Geometry: final body of the model. Coordinates: model frame, mm. Face numbers are marked on the shaded views. A direction names the side the tool comes from. Give positions to 0.01 mm unless a question says otherwise; leave off trailing zeros. Loops run counter-clockwise (first coordinate to the right, second up) from the corner with the lowest first, then second, coordinate; pieces in that order, holes last. Notation, with made-up numbers: (-23, 52) -> (-3, 52) arc R9 ccw to (-3, 62) -> close; hole circle Ø5 at (66, 4). An arc over 180 degrees is marked (long way). One line per question, with ' | ' between items. Start each with the question number.
Item 1: Mould query, pull axis Y, two halves, no side actions, for the marked faces 6, 7, 8 and 9. Classes: released by +Y, released by -Y, zero draft, split by the parting line, or undercut.
Item 2: Section A-A on x = 9.75. Return loops of the section in (y, z).
Item 3: Section B-B on y = 21. Return loops of the section in (x, z).
Item 4: Section D-D on x = 16.25. Give the number of separate pieces and of enclosed holes in the cut face, then the cut area to 3 significant figures.
Item 5: Set-up query: the marked faces 1, 2, 3, 4 and 5. Return all of +Z, -Z, +X, -X, +Y, -Y with unobstructed straight access to the full face (end or side cutting, diameter ignored); none if empty.
Item 6: Material intervals for line 1 along Z through (x, y) = (19, -15.5); line 2 along Z through (x, y) = (13.25, 0); line 3 along X through (y, z) = (9.5, 17), sorted ascending. Write a range as [from, to].
Item 7: Section C-C on x = 13.5. Return loops of the section in (y, z).
Item 8: Pin query (flat end, axial travel): P1, Ø0.7, axis at x = 7, y = 6, coming from the +Z side; P2, Ø1.5, axis at x = 5, z = 8.5, coming from the +Y side; P3, Ø3, axis at x = 5, z = 8, coming from the +Y side. Return the tip coordinate at first contact, or that it passes through.
from build123d import *

# Parameters (mm, degrees)
SKETCH1_R                = 10
BOSS_EXTRUDE2_DEPTH      = 20
SKETCH5_R                = 12
BOSS_EXTRUDE3_DEPTH      = 12
BOSS_EXTRUDE4_DEPTH      = 5
FILLET2_R                = 3.175
F_5_0_5_DIAMETER_HOLE1_D = 5
FILLET1_START            = 15.0000001
FILLET1_DEPTH            = 4.9999999
FILLET1_START_2          = 11.8249999
FILLET1_2_DEPTH          = 3.1750001
CIRPATTERN6_START        = 11.8249999
CIRPATTERN6_OUTLINE_R    = 2.5
CIRPATTERN6_DEPTH        = 8.1750001
SKETCH2_R                = 5.5
SHAFT_HOLE_DEPTH         = 41.025175904
SKETCH3_W                = 4
SKETCH3_H                = 3.6
KEYWAY_DEPTH             = 41.025175904


with BuildPart() as part:
    # Sketch1 → Boss-Extrude2 (new body)
    with BuildSketch(Plane(origin=(0, 0, 0), x_dir=(0, 0, -1), z_dir=(1, 0, 0))):
        Circle(SKETCH1_R)
    extrude(amount=BOSS_EXTRUDE2_DEPTH)

    # Sketch5 → Boss-Extrude3 (add)
    with BuildSketch(Plane.ZY.offset(-20)):
        Circle(SKETCH5_R)
    extrude(amount=BOSS_EXTRUDE3_DEPTH)

    # Sketch6 → Boss-Extrude4 (add)
    with BuildSketch(Plane(origin=(20, 0, 0), x_dir=(0, 0, -1), z_dir=(1, 0, 0))):
        with BuildLine():
            Line((-5, 20), (-5, 0))
            Line((-5, 0), (5, 0))
            Line((5, 0), (5, 20))
            ThreePointArc((5, 20), (0, 25), (-5, 20))
        make_face()
    extrude(amount=-BOSS_EXTRUDE4_DEPTH)

    # Fillet2
    fillet2_edges = [part.edges().sort_by_distance(p)[0] for p in [
        (15, 12, 0),
    ]]
    fillet(fillet2_edges, radius=FILLET2_R)

    # Ø5.0 (5) Diameter Hole1 (through all)
    with Locations(Plane(origin=(20, 0, 0), x_dir=(0, 0, -1), z_dir=(1, 0, 0))):
        with Locations((0, 20)):
            Hole(F_5_0_5_DIAMETER_HOLE1_D / 2)

    # Fillet1: read off the stored shape, not the designer's step
    # Fillet1 outline → Fillet1 (add)
    with BuildSketch(Plane.YZ.offset(FILLET1_START)):
        with BuildLine():
            ThreePointArc((9.921567416, -6.75), (11.357927862, -5.464466094), (13.228756555, -5))
            Line((13.228756555, -5), (10.908712115, -5))
            ThreePointArc((10.908712115, -5), (10.451830526, -5.895696622), (9.921567416, -6.75))
        make_face()
        with BuildLine():
            ThreePointArc((13.228756555, 5), (11.357927862, 5.464466094), (9.921567416, 6.75))
            ThreePointArc((9.921567416, 6.75), (10.451830526, 5.895696622), (10.908712115, 5))
            Line((10.908712115, 5), (13.228756555, 5))
        make_face()
    extrude(amount=FILLET1_DEPTH)

    # Fillet1 2 outline → Fillet1 2 (add)
    with BuildSketch(Plane.YZ.offset(FILLET1_START_2)):
        with BuildLine():
            ThreePointArc((9.921567416, -6.75), (11.357927862, -5.464466094), (13.228756555, -5))
            Line((13.228756555, -5), (10.908712115, -5))
            ThreePointArc((10.908712115, -5), (10.451830526, -5.895696622), (9.921567416, -6.75))
        make_face()
        with BuildLine():
            ThreePointArc((13.228756555, 5), (11.357927862, 5.464466094), (9.921567416, 6.75))
            ThreePointArc((9.921567416, 6.75), (10.451830526, 5.895696622), (10.908712115, 5))
            Line((10.908712115, 5), (13.228756555, 5))
        make_face()
    extrude(amount=FILLET1_2_DEPTH)

    # Fillet1 3 outline → Fillet1 3 (revolve, cut)
    with BuildSketch(Plane.YX):
        with BuildLine():
            Line((15.175, 11.8249999), (15.175, 15))
            ThreePointArc((15.175, 15), (12.92993597, 14.07006403), (12, 11.825))
            Line((12, 11.825), (15.175, 11.8249999))
        make_face()
    revolve(axis=Axis((0, 0, 0), (1, 0, 0)), mode=Mode.SUBTRACT)

    # CirPattern6: read off the stored shape, not the designer's step
    # CirPattern6 outline → CirPattern6 (add)
    # profile 1 of 4: a face of its own
    with BuildSketch(Plane.YZ.offset(CIRPATTERN6_START)):
        with BuildLine():
            Line((8.843193172, 11.036210153), (10.935622469, 17.476045354))
            ThreePointArc((10.935622469, 17.476045354), (7.725424859, 23.776412907), (1.425057306, 20.566215298))
            Line((1.425057306, 20.566215298), (-0.667371991, 14.126380096))
            ThreePointArc((-0.667371991, 14.126380096), (-1.687223357, 12.490644193), (-3.353698542, 11.521836055))
            ThreePointArc((-3.353698542, 11.521836055), (3.708203933, 11.412678195), (9.485564428, 7.350106631))
            ThreePointArc((9.485564428, 7.350106631), (8.706808817, 9.113418416), (8.843193172, 11.036210153))
        make_face()
        with Locations((6.180339887, 19.021130326)):
            Circle(CIRPATTERN6_OUTLINE_R, mode=Mode.SUBTRACT)
    # profile 2 of 4: a face of its own
    with BuildSketch(Plane.YZ.offset(CIRPATTERN6_START)):
        with BuildLine():
            ThreePointArc((-11.994267104, 0.370886295), (-9.708203933, 7.053423027), (-4.059166198, 11.292615719))
            ThreePointArc((-4.059166198, 11.292615719), (-5.976824079, 11.096868429), (-7.763362606, 11.820752981))
            Line((-7.763362606, 11.820752981), (-13.241413626, 15.800790018))
            ThreePointArc((-13.241413626, 15.800790018), (-20.225424859, 14.694631307), (-19.119266149, 7.710620074))
            Line((-19.119266149, 7.710620074), (-13.641215129, 3.730583038))
            ThreePointArc((-13.641215129, 3.730583038), (-12.400689243, 2.255176559), (-11.994267104, 0.370886295))
        make_face()
        with Locations((-16.180339887, 11.755705046)):
            Circle(CIRPATTERN6_OUTLINE_R, mode=Mode.SUBTRACT)
    # profile 3 of 4: a face of its own
    with BuildSketch(Plane.YZ.offset(CIRPATTERN6_START)):
        with BuildLine():
            ThreePointArc((8.843193172, -11.036210153), (8.706808817, -9.113418416), (9.485564428, -7.350106631))
            ThreePointArc((9.485564428, -7.350106631), (3.708203933, -11.412678195), (-3.353698542, -11.521836055))
            ThreePointArc((-3.353698542, -11.521836055), (-1.687223357, -12.490644193), (-0.667371991, -14.126380096))
            Line((-0.667371991, -14.126380096), (1.425057306, -20.566215298))
            ThreePointArc((1.425057306, -20.566215298), (7.725424859, -23.776412907), (10.935622469, -17.476045354))
            Line((10.935622469, -17.476045354), (8.843193172, -11.036210153))
        make_face()
        with Locations((6.180339887, -19.021130326)):
            Circle(CIRPATTERN6_OUTLINE_R, mode=Mode.SUBTRACT)
    # profile 4 of 4: a face of its own
    with BuildSketch(Plane.YZ.offset(CIRPATTERN6_START)):
        with BuildLine():
            ThreePointArc((-4.059166198, -11.292615719), (-9.708203933, -7.053423027), (-11.994267104, -0.370886295))
            ThreePointArc((-11.994267104, -0.370886295), (-12.400689243, -2.255176559), (-13.641215129, -3.730583038))
            Line((-13.641215129, -3.730583038), (-19.119266149, -7.710620074))
            ThreePointArc((-19.119266149, -7.710620074), (-20.225424859, -14.694631307), (-13.241413626, -15.800790018))
            Line((-13.241413626, -15.800790018), (-7.763362606, -11.820752981))
            ThreePointArc((-7.763362606, -11.820752981), (-5.976824079, -11.096868429), (-4.059166198, -11.292615719))
        make_face()
        with Locations((-16.180339887, -11.755705046)):
            Circle(CIRPATTERN6_OUTLINE_R, mode=Mode.SUBTRACT)
    extrude(amount=CIRPATTERN6_DEPTH)

    # CirPattern6 2 outline → CirPattern6 2 (revolve, cut)
    with BuildSketch(Plane.YX):
        with BuildLine():
            Line((25, 15), (15.175, 15))
            ThreePointArc((15.175, 15), (12.92993597, 14.07006403), (12, 11.825))
            Line((12, 11.825), (25, 11.8249999))
            Line((25, 11.8249999), (25, 15))
        make_face()
    revolve(axis=Axis((0, 0, 0), (1, 0, 0)), mode=Mode.SUBTRACT)

    # Sketch2 → Shaft hole (cut, through all)
    with BuildSketch(Plane.ZY):
        Circle(SKETCH2_R)
    extrude(amount=-SHAFT_HOLE_DEPTH, mode=Mode.SUBTRACT)

    # Sketch3 → Keyway (cut, through all)
    with BuildSketch(Plane.ZY):
        with Locations((0, 5.5)):
            Rectangle(SKETCH3_W, SKETCH3_H)
    extrude(amount=-KEYWAY_DEPTH, mode=Mode.SUBTRACT)


solid = part.part
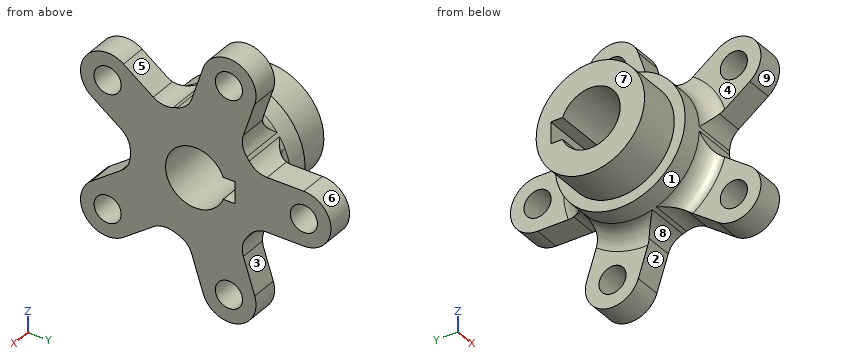
Result sheet:
1) face 6: released by +Y | face 7: zero draft | face 8: undercut | face 9: undercut
2) outline: circle Ø24 at (0, 0); hole (5.12, -2) -> (7.3, -2) -> (7.3, 2) -> (5.12, 2) arc R5.5 ccw (long way) to start
3) outline: (15, -4.9) -> (20, -4.9) -> (20, -2.29) -> (15, -2.29) -> close; (15, 2.29) -> (20, 2.29) -> (20, 4.9) -> (15, 4.9) -> close
4) separate pieces: 1 | enclosed holes: 6 | area: 874 mm²
5) face 1: -X | face 2: -Z, +X, -X | face 3: +X, -X, +Y | face 4: +Z, -X, -Y | face 5: +Z, +X, -X
6) line 1: z = [-16.71, -14.16], [-9.35, -5.08], [5.08, 9.35], [14.16, 16.71] | line 2: z = [-12.34, -5.5], [5.5, 12.34] | line 3: x = [15, 20]
7) outline: (-12.31, -2.05) arc R12.48 ccw to (-5.75, -11.07) arc R4 cw to (-4.06, -11.29) arc R12 ccw to (-3.35, -11.52) arc R4 cw to (-1.85, -12.34) arc R12.48 ccw to (8.75, -8.89) arc R4 cw to (9.49, -7.35) arc R12 ccw to (9.92, -6.75) arc R4 cw to (11.16, -5.57) arc R12.48 ccw to (11.16, 5.57) arc R4 cw to (9.92, 6.75) arc R12 ccw to (9.49, 7.35) arc R4 cw to (8.75, 8.89) arc R12.48 ccw to (-1.85, 12.34) arc R4 cw to (-3.35, 11.52) arc R12 ccw to (-4.06, 11.29) arc R4 cw to (-5.75, 11.07) arc R12.48 ccw to (-12.31, 2.05) arc R4 cw to (-11.99, 0.37) arc R12 ccw to (-11.99, -0.37) arc R4 cw to start; hole (5.12, -2) -> (7.3, -2) -> (7.3, 2) -> (5.12, 2) arc R5.5 ccw (long way) to start
8) P1: stops at z = 8.25 | P2: stops at y = 6.32 | P3: stops at y = 7.6
